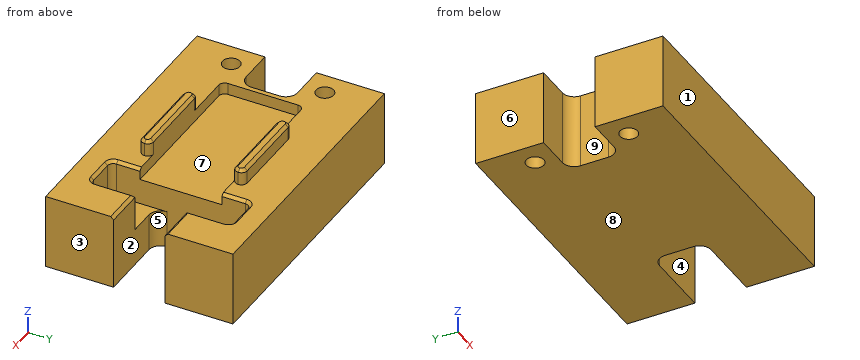
```python
from build123d import *

# Parameters (mm, degrees)
SKETCH1_W           = 50.8
SKETCH1_H           = 76.2
BOSS_EXTRUDE1_DEPTH = 13.97
SKETCH2_W           = 76.2
SKETCH2_H           = 50.8
BOSS_EXTRUDE2_DEPTH = 6.35
CUT_EXTRUDE1_DEPTH  = 10.16
SKETCH4_W           = 12.7
SKETCH4_H           = 13.97
SKETCH4_W_2         = 20.955
CUT_EXTRUDE2_DEPTH  = 51.096630625
SKETCH8_R           = 2.38125
CUT_EXTRUDE4_DEPTH  = 51.096630625
SKETCH10_W          = 23.749
SKETCH10_H          = 3.175
BOSS_EXTRUDE4_DEPTH = 4.318
SKETCH11_W          = 41.275
SKETCH11_H          = 22.225
CUT_EXTRUDE5_DEPTH  = 3.175
FILLET2_R           = 3.175
FILLET3_R           = 1.5875
CHAMFER3_SIZE       = 0.7874


with BuildPart() as part:
    # Sketch1 → Boss-Extrude1 (new body)
    with BuildSketch(Plane(origin=(0, 0, 0), x_dir=(0, 1, 0), z_dir=(0, 0, 1))):
        Rectangle(SKETCH1_W, SKETCH1_H)
    extrude(amount=-BOSS_EXTRUDE1_DEPTH)

    # Sketch2 → Boss-Extrude2 (add)
    with BuildSketch(Plane.XY):
        Rectangle(SKETCH2_W, SKETCH2_H)
    extrude(amount=BOSS_EXTRUDE2_DEPTH)

    # Sketch3 → Cut-Extrude1 (cut)
    with BuildSketch(Plane.XY.offset(6.35)):
        Polygon((38.1, 6.985), (38.1, -6.985), (27.305, -6.985), (27.305, -19.05), (17.145, -19.05), (17.145, 19.05), (27.305, 19.05), (27.305, 6.985), align=None)
    extrude(amount=-CUT_EXTRUDE1_DEPTH, mode=Mode.SUBTRACT)

    # Sketch4 → Cut-Extrude2 (cut, through all)
    with BuildSketch(Plane.XY.offset(6.35)):
        with Locations((-31.75, 0)):
            Rectangle(SKETCH4_W, SKETCH4_H)
        with Locations((27.6225, 0)):
            Rectangle(SKETCH4_W_2, SKETCH4_H)
    extrude(amount=-CUT_EXTRUDE2_DEPTH, mode=Mode.SUBTRACT)

    # Sketch8 → Cut-Extrude4 (cut, through all)
    with BuildSketch(Plane.XY.offset(6.35)):
        with Locations((-31.75, 12.7)):
            Circle(SKETCH8_R)
        with Locations((-31.75, -12.7)):
            Circle(SKETCH8_R)
    extrude(amount=-CUT_EXTRUDE4_DEPTH, mode=Mode.SUBTRACT)

    # Sketch10 → Boss-Extrude4 (add)
    with BuildSketch(Plane.XY.offset(6.35)):
        with Locations((0, 12.7)):
            Rectangle(SKETCH10_W, SKETCH10_H)
    boss_extrude4 = extrude(amount=BOSS_EXTRUDE4_DEPTH)

    # Sketch11 → Cut-Extrude5 (cut)
    with BuildSketch(Plane.XY.offset(6.35)):
        with Locations((-3.4925, 0)):
            Rectangle(SKETCH11_W, SKETCH11_H)
    extrude(amount=-CUT_EXTRUDE5_DEPTH, mode=Mode.SUBTRACT)

    # Mirror1: Boss-Extrude4 across plane
    add(boss_extrude4.mirror(Plane.ZX))

    # Fillet2
    fillet2_edges = [part.edges().sort_by_distance(p)[0] for p in [
        (-25.4, 6.985, -3.81),
        (-25.4, -6.985, -3.81),
        (17.145, -6.985, -8.89),
        (17.145, 6.985, -8.89),
    ]]
    fillet(fillet2_edges, radius=FILLET2_R)

    # Fillet3
    fillet3_edges = [part.edges().sort_by_distance(p)[0] for p in [
        (-24.13, -11.1125, 4.7625),
        (-24.13, 11.1125, 4.7625),
        (17.145, -19.05, 1.27),
        (27.305, -19.05, 1.27),
        (11.8745, 14.2875, 8.509),
        (11.8745, -11.1125, 8.509),
        (11.8745, -14.2875, 8.509),
        (11.8745, 11.1125, 8.509),
        (17.145, 19.05, 1.27),
        (-11.8745, -14.2875, 8.509),
        (-11.8745, -11.1125, 8.509),
        (-11.8745, 11.1125, 8.509),
        (-11.8745, 14.2875, 8.509),
        (27.305, 19.05, 1.27),
    ]]
    fillet(fillet3_edges, radius=FILLET3_R - 0.0001)  # a hair under: the kernel refuses the full size

    # Chamfer3
    chamfer3_edges = [part.edges().sort_by_distance(p)[0] for p in [
        (17.145, -14.28755, 6.35),
        (0, -11.1125, 10.668),
        (0, 11.1125, 10.668),
        (22.225, -19.05, 6.35),
        (17.145, 14.28755, 6.35),
        (27.305, -12.2238, 6.35),
        (0, 14.2875, 10.668),
        (-11.409561304, 13.822561304, 10.668),
        (-11.409561304, 11.577438696, 10.668),
        (11.409561304, 11.577438696, 10.668),
        (11.409561304, 13.822561304, 10.668),
        (0, -14.2875, 10.668),
        (-11.409561304, -11.577438696, 10.668),
        (-11.409561304, -13.822561304, 10.668),
        (11.409561304, -13.822561304, 10.668),
        (11.409561304, -11.577438696, 10.668),
        (22.225, 19.05, 6.35),
        (17.609938696, -18.585061304, 6.35),
        (26.840061304, -18.585061304, 6.35),
        (17.609938696, 18.585061304, 6.35),
        (26.840061304, 18.585061304, 6.35),
        (32.7025, -6.985, 6.35),
        (32.7025, 6.985, 6.35),
        (27.305, 12.2238, 6.35),
    ]]
    chamfer(chamfer3_edges, length=CHAMFER3_SIZE)


solid = part.part
```
Input: part model. Units: mm. Frame: model coordinates. Face numbers are marked on the shaded views. A direction names the side the tool comes from. Give positions to 0.01 mm unless a question says otherwise; leave off trailing zeros. Order: outer loops, then holes, each group sorted by start corner. A loop starts at its lowest first (then second) coordinate and runs counter-clockwise, first axis right, second up. Notation, with made-up numbers: (-3, 56.25) - (30, 56.25) arc R17 cw to (30, 61.25) - close; hole circle Ø5 at (-11, -4.75). An arc over 180 degrees is marked (long way). Use a Markdown table: item, result.
(1) Pin query (flat end, axial travel): pin 1 (4 mm diameter, centred on x = -15.5, y = -2.5, fed in from +Z) (3 decimals); pin 2 (11 mm diameter, centred on x = 23.5, y = 13.5, fed in from +Z); pin 3 (6 mm diameter, centred on x = -31.75, y = -12.7, fed in from +Z). Return the tip coordinate at first contact, or that it passes through.
Computed values:
| item | result |
|---|---|
| pin 1 | stops at z = 3.175 |
| pin 2 | stops at z = 6.35 |
| pin 3 | stops at z = 6.35 |
(2) Access query for the marked faces 5, 6, 7, 8 and 9. Directions: +Z, -Z, +X, -X, +Y, -Y. A direction counts if a zero-diameter tool reaches every point of the face in a straight line with its end or side. Return the directions, or none.
Computed values:
| item | result |
|---|---|
| face 5 | +Z, -Z, +X |
| face 6 | +Z, -Z, -X, +Y, -Y |
| face 7 | +Z |
| face 8 | -Z, +X, -X, +Y, -Y |
| face 9 | +Z, -Z, -X |
(3) Line query: line 1 (Y direction, x = -31.75, z = -4.5) (3 decimals); line 2 (X direction, y = 12.5, z = 3) (3 decimals); line 3 (Y direction, x = -3.5, z = 7.75). Output: solid intervals per line, ascending. Write a range as from..to.
Computed values:
| item | result |
|---|---|
| line 1 | y = -25.4..-15.081, -10.319..-6.985, 6.985..10.319, 15.081..25.4 |
| line 2 | x = -38.1..-34.123, -29.377..17.145, 27.305..38.1 |
| line 3 | y = -14.29..-11.11, 11.11..14.29 |
(4) Draft query along Y for the marked faces 1, 2, 3 and 4. Return one class per face: released by +Y, released by -Y, zero draft, split by the parting line, or undercut.
Computed values:
| item | result |
|---|---|
| face 1 | released by -Y |
| face 2 | undercut |
| face 3 | zero draft |
| face 4 | undercut |
(5) Section query A-A (x = 24.5). Output: boundary loops of the cut face in (y, z) (3 decimals).
Computed values:
| item | result |
|---|---|
| outline | (-25.4, -13.97) - (-6.985, -13.97) - (-6.985, -3.81) - (-19.05, -3.81) - (-19.05, 5.563) - (-19.837, 6.35) - (-25.4, 6.35) - close; (6.985, -13.97) - (25.4, -13.97) - (25.4, 6.35) - (19.837, 6.35) - (19.05, 5.563) - (19.05, -3.81) - (6.985, -3.81) - close |
(6) Section query C-C (x = -31.75). Output: boundary loops of the cut face in (y, z) (3 decimals).
Computed values:
| item | result |
|---|---|
| outline | (-25.4, -13.97) - (-15.081, -13.97) - (-15.081, 6.35) - (-25.4, 6.35) - close; (-10.319, -13.97) - (-6.985, -13.97) - (-6.985, 6.35) - (-10.319, 6.35) - close; (6.985, -13.97) - (10.319, -13.97) - (10.319, 6.35) - (6.985, 6.35) - close; (15.081, -13.97) - (25.4, -13.97) - (25.4, 6.35) - (15.081, 6.35) - close |
(7) Section query B-B (z = 1.5). State how many separate pieces and enclosed holes the cut face has, then the cut area to 3 significant figures.
Computed values:
| item | result |
|---|---|
| separate pieces | 1 |
| enclosed holes | 2 |
| area | 3,130 mm2 |
